Build history of the part. All positions in model axes, mm. Face numbers are marked on the shaded views. A direction names the side the tool comes from. Coordinates: 2 decimals unless noted, no trailing zeros. Loops run counter-clockwise (first coordinate to the right, second up) from the corner with the lowest first, then second, coordinate; pieces in that order, holes last.
(1) Tool access for the marked faces 4, 5, 6, 7 and 8: list every direction of +Z, -Z, +X, -X, +Y, -Y with a clear straight run to the whole face (end or side of a thin tool).
(2) Slice it at D-D (y = 2.85). Give the cut face in (x, z).
(3) Slice it at C-C (z = 0.8). Give the cut face in (x, y), and give its area (3 significant figures).
(4) Slice it at B-B (y = 1.7). Give the cut face in (x, z) (3 decimals), and give its area (3 significant figures).
(5) Slice it at A-A (x = 0.7). Give the cut face in (y, z) (3 decimals).
(6) Wall check: L1, parallel to Y at x = 5.7, z = 3.15 (3 decimals); L2, parallel to Y at x = 5.7, z = 2.6 (3 decimals); L3, parallel to X at y = 0.6, z = 1.35. Give the ranges that are in metal, low to high.
(7) Two-plate mould, pull along Y, no slides. Class the marked faces 1, 2 and 3: pulls with the +Y half, pulls with the -Y half, needs draft (parallel to the pull), parting line crosses it, or undercut.
(8) Flat gauge pins, fed straight in: P1, Ø1.5, axis at x = 5.7, y = 1.7, coming from the +Z side; P2, Ø1.4, axis at y = 3.5, z = 2.5, coming from the +X side; P3, Ø2, axis at x = 3.5, z = 2.5, coming from the -Y side; P4, Ø1.5, axis at x = 5.5, z = 2, coming from the -Y side. Where does each tip first touch, or does it go through?
from build123d import *

# Parameters (mm, degrees)
SKETCH1_W           = 6.8
SKETCH1_H           = 5
BOSS_EXTRUDE1_DEPTH = 3.8
SKETCH3_W           = 2.8
SKETCH3_H           = 2.9
CUT_EXTRUDE2_DEPTH  = 10.340235543
SKETCH4_W           = 1.9
SKETCH4_H           = 0.2
CUT_EXTRUDE3_DEPTH  = 2.2
HOLE1_D             = 1.05
HOLE1_CBORE_D       = 1.3
HOLE1_CBORE_DEPTH   = 1.2
CUT_EXTRUDE9_DEPTH  = 10.340235543
CUT_EXTRUDE10_DEPTH = 0.3
SKETCH20_W          = 5
SKETCH20_H          = 1.3
CUT_EXTRUDE11_DEPTH = 0.3


with BuildPart() as part:
    # Sketch1 → Boss-Extrude1 (new body)
    with BuildSketch(Plane(origin=(0, 4, 0), x_dir=(-1, 0, 0), z_dir=(0, 1, 0))):
        with Locations((-3.4, 2.5)):
            Rectangle(SKETCH1_W, SKETCH1_H)
    extrude(amount=-BOSS_EXTRUDE1_DEPTH)

    # Sketch3 → Cut-Extrude2 (cut, through all)
    with BuildSketch(Plane.XY.offset(5)):
        with Locations((3.2, 1.65)):
            Rectangle(SKETCH3_W, SKETCH3_H)
    extrude(amount=-CUT_EXTRUDE2_DEPTH, mode=Mode.SUBTRACT)

    # Sketch4 → Cut-Extrude3 (cut)
    with BuildSketch(Plane(origin=(6.8, 0, 0), x_dir=(0, 0, -1), z_dir=(1, 0, 0))):
        with Locations((-1.9, 0.3)):
            Rectangle(SKETCH4_W, SKETCH4_H)
    extrude(amount=-CUT_EXTRUDE3_DEPTH, mode=Mode.SUBTRACT)

    # Hole1 (through all)
    with Locations(Plane(origin=(0, 0, 0), x_dir=(-1, 0, 0), z_dir=(0, 0, -1))):
        with Locations((-5.7, 1.7), (-0.7, 1.7)):
            CounterBoreHole(HOLE1_D / 2, HOLE1_CBORE_D / 2, HOLE1_CBORE_DEPTH)

    # Sketch18 → Cut-Extrude9 (cut, through all)
    with BuildSketch(Plane(origin=(6.8, 0, 0), x_dir=(0, 0, -1), z_dir=(1, 0, 0))):
        Polygon((-1.288675135, 4), (-3.711324865, 4), (-4, 3.5), (-1, 3.5), align=None)
    extrude(amount=-CUT_EXTRUDE9_DEPTH, mode=Mode.SUBTRACT)

    # Sketch19 → Cut-Extrude10 (cut)
    with BuildSketch(Plane(origin=(0, 3.5, 0), x_dir=(1, 0, 0), z_dir=(0, 1, 0))):
        with BuildLine():
            Line((6.8, -1.75), (6, -1.75))
            ThreePointArc((6, -1.75), (6.530330086, -1.969669914), (6.75, -2.5))
            ThreePointArc((6.75, -2.5), (6.530330086, -3.030330086), (6, -3.25))
            Line((6, -3.25), (6.8, -3.25))
            Line((6.8, -3.25), (6.8, -1.75))
        make_face()
        with BuildLine():
            ThreePointArc((6.75, -2.5), (6.530330086, -1.969669914), (6, -1.75))
            Line((6, -1.75), (6, -3.25))
            ThreePointArc((6, -3.25), (6.530330086, -3.030330086), (6.75, -2.5))
        make_face()
        with BuildLine():
            Line((6, -3.25), (6, -1.75))
            ThreePointArc((6, -1.75), (5.25, -2.5), (6, -3.25))
        make_face()
    extrude(amount=-CUT_EXTRUDE10_DEPTH, mode=Mode.SUBTRACT)

    # Sketch20 → Cut-Extrude11 (cut)
    with BuildSketch(Plane(origin=(6.8, 0, 0), x_dir=(0, 0, -1), z_dir=(1, 0, 0))):
        with Locations((-2.5, 3.35)):
            Rectangle(SKETCH20_W, SKETCH20_H)
    extrude(amount=-CUT_EXTRUDE11_DEPTH, mode=Mode.SUBTRACT)


solid = part.part
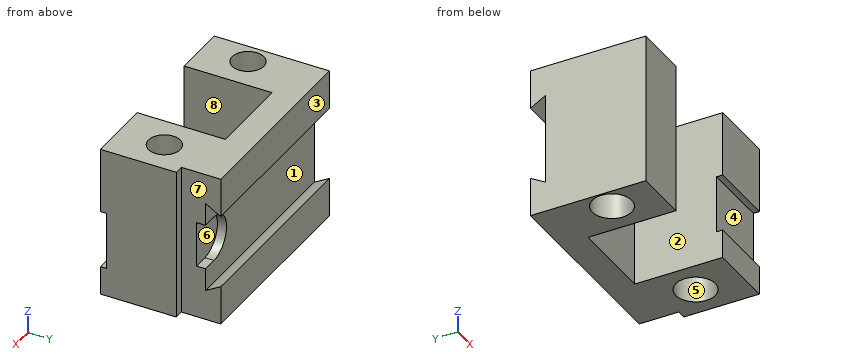
Response values:
1. face 4: +X, -Y
1. face 5: -Z
1. face 6: +X, +Y
1. face 7: +Z, -Z, +X, +Y
1. face 8: +Z, -Z, -Y
2. outline: (0, 0) - (1.8, 0) - (1.8, 5) - (0, 5) - close; (4.6, 0) - (6.5, 0) - (6.5, 5) - (4.6, 5) - close
3. outline: (0, 0.2) - (1.8, 0.2) - (1.8, 3.1) - (4.6, 3.1) - (4.6, 0.2) - (6.8, 0.2) - (6.8, 2.7) - (6.5, 2.7) - (6.5, 4) - (0, 4) - close; hole circle Ø1.3 at (0.7, 1.7); hole circle Ø1.3 at (5.7, 1.7)
3. area: 14.7 mm2
4. outline: (0, 0) - (0.05, 0) - (0.05, 1.2) - (0.175, 1.2) - (0.175, 5) - (0, 5) - close; (1.225, 1.2) - (1.35, 1.2) - (1.35, 0) - (1.8, 0) - (1.8, 5) - (1.225, 5) - close; (4.6, 0) - (5.05, 0) - (5.05, 1.2) - (5.175, 1.2) - (5.175, 5) - (4.6, 5) - close; (6.225, 1.2) - (6.35, 1.2) - (6.35, 0) - (6.8, 0) - (6.8, 5) - (6.225, 5) - close
4. area: 8.90 mm2
5. outline: (0.2, 0) - (1.05, 0) - (1.05, 1.2) - (1.175, 1.2) - (1.175, 5) - (0.2, 5) - close; (2.225, 1.2) - (2.35, 1.2) - (2.35, 0) - (4, 0) - (4, 1.289) - (3.5, 1) - (3.5, 4) - (4, 3.711) - (4, 5) - (2.225, 5) - close
6. L1: y = 0.2 to 1.175, 2.225 to 3.2
6. L2: y = 0.4 to 1.175, 2.225 to 3.2
6. L3: x = 0 to 1.8, 4.6 to 6.8
7. face 1: undercut
7. face 2: needs draft
7. face 3: pulls with the +Y half
8. P1: stops at z = 5
8. P2: stops at x = 6.5
8. P3: stops at y = 3.1
8. P4: stops at y = 0.4
